from build123d import *

# Parameters (mm, degrees)
F1_DEPTH = 17
F2_R     = 2.6
F3_DEPTH = 3.4
F4_DEPTH = 9.001


# Not quite as in the source:
# - ends of sketch curves that miss each other by under 0.0002 mm in the source are joined


with BuildPart() as f1:
    # F0 (on Front) → F1 (new body)
    with BuildSketch(Plane.XZ):
        with BuildLine():
            ThreePointArc((-8.4332967812, 5.0428927812), (-8.6500695325, 4.7184694324), (-8.72619, 4.335786))
            Line((-8.72619, 4.335786), (-8.72619, -4.835786))
            ThreePointArc((-8.72619, -4.835786), (-8.6500695325, -5.2184694324), (-8.4332967812, -5.5428927812))
            Line((-8.4332967812, -5.5428927812), (-5.519083, -8.457107))
            ThreePointArc((-5.519083, -8.457107), (-5.1946594324, -8.6738795325), (-4.811976, -8.75))
            Line((-4.811976, -8.75), (-3.72619, -8.75))
            ThreePointArc((-3.72619, -8.75), (-3.0190832188, -8.4571067812), (-2.72619, -7.75))
            Line((-2.72619, -7.75), (-2.72619, -5.15))
            Line((-2.72619, -5.15), (0.27381, -5.15))
            Line((0.27381, -5.15), (0.27381, 4.65))
            Line((0.27381, 4.65), (-2.72619, 4.65))
            Line((-2.72619, 4.65), (-2.72619, 7.25))
            ThreePointArc((-2.72619, 7.25), (-3.0190832188, 7.9571067812), (-3.72619, 8.25))
            Line((-3.72619, 8.25), (-4.811976, 8.25))
            ThreePointArc((-4.811976, 8.25), (-5.1946594324, 8.1738795325), (-5.5190827812, 7.9571067812))
            Line((-5.5190827812, 7.9571067812), (-8.4332967812, 5.0428927812))
        make_face()
    extrude(amount=-F1_DEPTH)

    # F2 (on face) → F3 (cut)
    with BuildSketch(Plane(origin=(-8.72619, 0, 0), x_dir=(0, -1, 0), z_dir=(-1, 0, 0))):
        Polygon((-11.6258979104, -4.835786), (-5.3741020896, -4.835786), (-2.7264973081, -0.25), (-5.3741020896, 4.335786), (-11.6258979104, 4.335786), (-14.2735026919, -0.25), align=None)
        with Locations((-8.5, -0.25)):
            Circle(F2_R, mode=Mode.SUBTRACT)
        with Locations((-8.5, -0.25)):
            Circle(F2_R)
    extrude(amount=-F3_DEPTH, mode=Mode.SUBTRACT)

    # F2 (on face) → F4 (cut, through all)
    with BuildSketch(Plane(origin=(-8.72619, 0, 0), x_dir=(0, -1, 0), z_dir=(-1, 0, 0))):
        with Locations((-8.5, -0.25)):
            Circle(F2_R)
    extrude(amount=-F4_DEPTH, mode=Mode.SUBTRACT)


solid = f1.part
Work out the finished part from the listing and answer in its coordinate system (mm). A direction names the side the tool comes from. Coordinates: 2 decimals unless noted, no trailing zeros. Loops run counter-clockwise (first coordinate to the right, second up) from the corner with the lowest first, then second, coordinate; pieces in that order, holes last. Notation, with made-up numbers: M -31,82.5 L 15,82.5 A18 ccw 15,105.5 Z; hole C 14.25,40.25 d2. An arc over 180 degrees is marked long. Answer in a Markdown table with one row per item. Add a question column.
1. Find section C-C, the plane y = 2.5. Write down the section's boundary in (x, z), then the cut area to 3 significant figures.
2. Find section D-D, the plane z = -1.25. Write down the section's boundary in (x, y).
3. A tool of negligible diameter and unlimited length cuts with its end or side. For faces 1 (the flat face through (-7.05, 4.069, -2.575)), 2 (the flat face through (0.274, 6, -2)), 3 (the flat face through (-1, 8, -5.15)), from which of +Z, -Z, +X, -X, +Y, -Y can it reach the whole face along a straight path? Write none if from no direction.
4. Flat-ended cylindrical pins translate along their axes: P1, Ø3, axis at y = 7.5, z = 6.5, coming from the +X side; P2, Ø1.5, axis at x = -1.5, y = 5.5, coming from the -Z side; P3, Ø0.9, axis at x = -1, y = 8, coming from the +Z side. Find the tip coordinate at first contact, or state that the pin passes through.
5. Find section A-A, the plane y = 7.5. Write down the section's boundary in (x, z), then the cut area to 3 significant figures.
6. Consider L1, parallel to Z at x = -1.45, y = 8.5; L2, parallel to X at y = 11.75, z = -3.5; L3, parallel to Z at x = -4, y = 8.5. Determine where each line is inside the solid, lowest interval first.
7. The mould has two halves that part along Z. Classify faces 4 (the flat face through (-2.726, 8, 6)), 5 (the flat face through (-7.05, 12.931, 2.075)), 6 (the flat face through (-6.997, 8.381, -6.98)), 7 (the flat face through (-7, 8, 4.336)): pulls with the +Z half, pulls with the -Z half, needs draft (parallel to the pull), parting line crosses it, or undercut.
8. Find section B-B, the plane z = 1. Write down the section's boundary in (x, y), then the cut area to 3 significant figures.
Reported:
| question | item | result |
|---|---|---|
| 1 | outline | M -8.73,-4.84 A1 ccw -8.43,-5.54 L -5.52,-8.46 A1 ccw -4.81,-8.75 L -3.73,-8.75 A1 ccw -2.73,-7.75 L -2.73,-5.15 L 0.27,-5.15 L 0.27,4.65 L -2.73,4.65 L -2.73,7.25 A1 ccw -3.73,8.25 L -4.81,8.25 A1 ccw -5.52,7.96 L -8.43,5.04 A1 ccw -8.73,4.34 Z |
| 1 | area | 119 mm^2 |
| 2 | outline | M -8.73,0 L 0.27,0 L 0.27,6.1 L -5.33,6.1 L -5.33,3.3 L -8.73,3.3 Z; M -8.73,13.7 L -5.33,13.7 L -5.33,10.9 L 0.27,10.9 L 0.27,17 L -8.73,17 Z |
| 3 | face 1 | -X |
| 3 | face 2 | +Z, -Z, +X, +Y, -Y |
| 3 | face 3 | -Z, +X, +Y, -Y |
| 4 | P1 | stops at x = -2.73 |
| 4 | P2 | stops at z = -5.15 |
| 4 | P3 | stops at z = 4.65 |
| 5 | outline | M -8.73,-4.84 A1 ccw -8.43,-5.54 L -5.52,-8.46 A1 ccw -4.81,-8.75 L -3.73,-8.75 A1 ccw -2.73,-7.75 L -2.73,-5.15 L 0.27,-5.15 L 0.27,-2.65 L -5.33,-2.65 L -5.33,-4.84 Z; M -8.73,4.34 L -5.33,4.34 L -5.33,2.15 L 0.27,2.15 L 0.27,4.65 L -2.73,4.65 L -2.73,7.25 A1 ccw -3.73,8.25 L -4.81,8.25 A1 ccw -5.52,7.96 L -8.43,5.04 A1 ccw Z |
| 5 | area | 60.6 mm^2 |
| 6 | L1 | z = -5.15 to -2.85, 2.35 to 4.65 |
| 6 | L2 | x = -5.33 to 0.27 |
| 6 | L3 | z = -8.75 to -2.85, 2.35 to 8.25 |
| 7 | face 4 | needs draft |
| 7 | face 5 | undercut |
| 7 | face 6 | pulls with the -Z half |
| 7 | face 7 | undercut |
| 8 | outline | M -8.73,0 L 0.27,0 L 0.27,6.22 L -5.33,6.22 L -5.33,3.45 L -8.73,3.45 Z; M -8.73,13.55 L -5.33,13.55 L -5.33,10.78 L 0.27,10.78 L 0.27,17 L -8.73,17 Z |
| 8 | area | 93.1 mm^2 |
